Here's how the part is built. I have some questions about the finished solid (model axes, mm). A direction names the side the tool comes from. Give positions to 0.01 mm unless a question says otherwise; leave off trailing zeros. Loops run counter-clockwise (first coordinate to the right, second up) from the corner with the lowest first, then second, coordinate; pieces in that order, holes last.
Q1. We'd pull the mould along Y, two halves only. Please class faces 4 (the face through (-187.95, 136.56, 0.14)), 5 (the face through (123.674, 167.646, 0.14)), 6 (the face through (-15, -30, 10)), 7 (the face through (-250.284, 100.97, 0.14)): +Y half, -Y half, draft (parallel to the pull), parting line (faces both ways), or undercut.
Q2. I need wall thicknesses on line 1 (X direction, y = 43, z = -3); line 2 (X direction, y = 23.5, z = 5.5); line 3 (Y direction, x = 1.5, z = 6). Which ranges of each line are inside material? Lowest first, please.
Q3. If we section it at C-C (y = -202): Please give me the cut outline in (x, z), plus the area to 3 significant figures.
Q4. If we section it at B-B (x = 206.5): Please give me the cut outline in (y, z).
Q5. For faces 1 (the face through (-130.8, -87.7, -0.1)), 2 (the face through (-63.95, 68.54, -0.14)), 3 (the face through (126.81, 158.15, -0.14)), which set-ups out of +Z, -Z, +X, -X, +Y, -Y let a thin tool reach every point of the face, with its end or its side?
Q6. If we section it at D-D (y = 27): Please give me the cut outline in (x, z).
Q7. Will these pins go through, and if not, where does the flat tip stop? P1, Ø8, axis at x = -182, z = 2.5, coming from the +Y side; P2, Ø5, axis at x = 99.5, z = -8, coming from the +Y side; P3, Ø3, axis at x = 83.5, z = -8, coming from the +Y side.
Q8. If we section it at A-A (z = 5): Please give me the cut outline in (x, y).
from build123d import *

# Parameters (mm, degrees)
CROQUIS3_W = 20
CROQUIS3_H = 10


with BuildPart() as part:
    # Barrer1: sweep along a path in Croquis2
    with BuildLine(Plane.XY) as barrer1_path:
        Line((-149.137435996, 156.432354984), (-225.686991426, 117.238406938))
        ThreePointArc((-225.686991426, 117.238406938), (-240.672072816, 98.182936179), (-235.950755595, 74.405367047))
        Line((-235.950755595, 74.405367047), (-12.549830507, -233.795760351))
        ThreePointArc((-12.549830507, -233.795760351), (0, -240.19896123), (12.549830507, -233.795760351))
        Line((12.549830507, -233.795760351), (235.950755595, 74.405367047))
        ThreePointArc((235.950755595, 74.405367047), (240.672072816, 98.182936179), (225.686991426, 117.238406938))
        Line((225.686991426, 117.238406938), (149.137435996, 156.432354984))
        ThreePointArc((149.137435996, 156.432354984), (126.505149479, 158.04802573), (109.636839036, 142.872687588))
        Line((109.636839036, 142.872687588), (35.347492768, -16.478918502))
        ThreePointArc((35.347492768, -16.478918502), (0, -39), (-35.347492768, -16.478918502))
        Line((-35.347492768, -16.478918502), (-109.636839036, 142.872687588))
        ThreePointArc((-109.636839036, 142.872687588), (-126.505149479, 158.04802573), (-149.137435996, 156.432354984))
    # Croquis3 → Barrer1 (sweep)
    with BuildSketch(Plane(origin=(0, 0, 0), x_dir=(0, 0, -1), z_dir=(1, 0, 0))):
        with Locations((0, -34)):
            Rectangle(CROQUIS3_W, CROQUIS3_H)
    sweep(path=barrer1_path.line)


solid = part.part
Check sheet entries:
1. face 4: undercut
1. face 5: +Y half
1. face 6: draft
1. face 7: parting line
2. line 1: x = -225.54 to -213.19, -63.08 to -52.04, 52.04 to 63.08, 213.19 to 225.54
2. line 2: x = -211.4 to -199.05, -53.99 to -42.95, 42.95 to 53.99, 199.05 to 211.4
2. line 3: y = -250.15 to -240.13, -38.97 to -28.96
3. outline: (-47.95, -10) - (-35.6, -10) - (-35.6, 10) - (-47.95, 10) - close; (35.6, -10) - (47.95, -10) - (47.95, 10) - (35.6, 10) - close
3. area: 494 mm2
4. outline: (16.74, -10) - (33.78, -10) - (33.78, 10) - (16.74, 10) - close; (127.06, -10) - (138.3, -10) - (138.3, 10) - (127.06, 10) - close
5. face 1: +Z, -Z, -X, -Y
5. face 2: +Z, -Z, +Y
5. face 3: +Z, -Z
6. outline: (-213.94, -10) - (-201.59, -10) - (-201.59, 10) - (-213.94, 10) - close; (-55.62, -10) - (-44.58, -10) - (-44.58, 10) - (-55.62, 10) - close; (44.58, -10) - (55.62, -10) - (55.62, 10) - (44.58, 10) - close; (201.59, -10) - (213.94, -10) - (213.94, 10) - (201.59, 10) - close
7. P1: stops at y = 152.89
7. P2: stops at y = 149.86
7. P3: stops at y = 113.69
8. outline: (-244.05, 68.54) - (-20.65, -239.66) arc R25.5 ccw to (20.65, -239.66) - (244.05, 68.54) arc R39 ccw to (230.24, 126.14) - (153.69, 165.33) arc R39 ccw to (100.57, 147.1) - (26.28, -12.25) arc R29 cw to (-26.28, -12.25) - (-100.57, 147.1) arc R39 ccw to (-153.69, 165.33) - (-230.24, 126.14) arc R39 ccw to start; hole (-235.95, 74.41) - (-12.55, -233.8) arc R15.5 ccw to (12.55, -233.8) - (235.95, 74.41) arc R29 ccw to (225.69, 117.24) - (149.14, 156.43) arc R29 ccw to (109.64, 142.87) - (35.35, -16.48) arc R39 cw to (-35.35, -16.48) - (-109.64, 142.87) arc R29 ccw to (-149.14, 156.43) - (-225.69, 117.24) arc R29 ccw to start
